Could you check a few things on this model? Use its own coordinates, in mm. Give positions to 0.01 mm unless a question says otherwise; leave off trailing zeros. Loops run counter-clockwise (first coordinate to the right, second up) from the corner with the lowest first, then second, coordinate; pieces in that order, holes last. Notation, with made-up numbers: M 12.5,-18.75 L 69.5,-18.75 A29 cw 69.5,1.25 Z; hole C -36.5,85 d3. An arc over 180 degrees is marked long. Return JSON: item names as keys, results as strings. Group by question number.
1. Please list where these lines run through material, in increasing order: line 1 (X direction, y = 2.35, z = 66); line 2 (X direction, y = 1.45, z = -13.5); line 3 (X direction, y = 1.45, z = 0).
2. If we section it at A-A (z = 30): Write out the boundary of the cut face in (x, y).
3. If we section it at C-C (y = 2.3): State how many separate pieces and enclosed holes the cut face has, plus the area to 3 significant figures.
4. For pin 1 (2.5 mm diameter, centred on x = 90, z = 0, fed in from +Y), with a flat end and sliding along its axis, tell me the tip position at first contact or that it passes through.
5. If we section it at B-B (x = -63.64): Write out the boundary of the cut face in (y, z), plus the area to 3 significant figures.
```python
from build123d import *

# Parameters (mm, degrees)
SKETCH_1_W          = 200
SKETCH_1_H          = 200
SKETCH_1_R          = 2
EXTRUDE_1_DEPTH     = 3
FILLET_1_R          = 25
CUT_EXTRUDE_1_DEPTH = 3


with BuildPart() as part:
    # Эскиз1 → Бобышка-Вытянуть1 (new body)
    with BuildSketch(Plane(origin=(0, 0, 0), x_dir=(1, 0, 0), z_dir=(0, 1, 0))):
        Rectangle(SKETCH_1_W, SKETCH_1_H)
        with Locations(Location((-90, 0, 0), (0, 0, 270))):
            Circle(SKETCH_1_R, mode=Mode.SUBTRACT)
        with Locations(Location((0, 90, 0), (0, 0, 270))):
            Circle(SKETCH_1_R, mode=Mode.SUBTRACT)
        with Locations(Location((90, 0, 0), (0, 0, 270))):
            Circle(SKETCH_1_R, mode=Mode.SUBTRACT)
        with Locations(Location((0, -90, 0), (0, 0, 270))):
            Circle(SKETCH_1_R, mode=Mode.SUBTRACT)
        with BuildLine():
            Line((-66.14, -76.211231978), (-66.14, 76.211231978))
            ThreePointArc((-66.14, 76.211231978), (-63.64, 78.711231978), (-61.14, 76.211231978))
            Line((-61.14, 76.211231978), (-61.14, -76.211231978))
            ThreePointArc((-61.14, -76.211231978), (-63.64, -78.711231978), (-66.14, -76.211231978))
        make_face(mode=Mode.SUBTRACT)
        with BuildLine():
            Line((66.14, -76.211231978), (66.14, 76.211231978))
            ThreePointArc((66.14, 76.211231978), (63.64, 78.711231978), (61.14, 76.211231978))
            Line((61.14, 76.211231978), (61.14, -76.211231978))
            ThreePointArc((61.14, -76.211231978), (63.64, -78.711231978), (66.14, -76.211231978))
        make_face(mode=Mode.SUBTRACT)
        with BuildLine():
            Line((1.5, 76.211231978), (1.5, 23.747339046))
            ThreePointArc((1.5, 23.747339046), (0, 22.247339046), (-1.5, 23.747339046))
            Line((-1.5, 23.747339046), (-1.5, 76.211231978))
            ThreePointArc((-1.5, 76.211231978), (0, 77.711231978), (1.5, 76.211231978))
        make_face(mode=Mode.SUBTRACT)
        with BuildLine():
            Line((1.5, -76.211231978), (1.5, -23.747339046))
            ThreePointArc((1.5, -23.747339046), (0, -22.247339046), (-1.5, -23.747339046))
            Line((-1.5, -23.747339046), (-1.5, -76.211231978))
            ThreePointArc((-1.5, -76.211231978), (0, -77.711231978), (1.5, -76.211231978))
        make_face(mode=Mode.SUBTRACT)
        with BuildLine():
            Line((-1.5, -9.644775033), (-1.5, 9.644775033))
            ThreePointArc((-1.5, 9.644775033), (0, 11.144775033), (1.5, 9.644775033))
            Line((1.5, 9.644775033), (1.5, -9.644775033))
            ThreePointArc((1.5, -9.644775033), (0, -11.144775033), (-1.5, -9.644775033))
        make_face(mode=Mode.SUBTRACT)
    extrude(amount=EXTRUDE_1_DEPTH)

    # Скругление1
    fillet_1_edges = [part.edges().sort_by_distance(p)[0] for p in [
        (100, 1.5, 100),
        (-100, 1.5, 100),
        (-100, 1.5, -100),
        (100, 1.5, -100),
    ]]
    fillet(fillet_1_edges, radius=FILLET_1_R)

    # Эскиз2 → Вырез-Вытянуть1 (cut)
    with BuildSketch(Plane(origin=(0, 3, 0), x_dir=(1, 0, 0), z_dir=(0, 1, 0))):
        with BuildLine():
            Line((51.61254098, 2.5), (75.66745902, 2.5))
            ThreePointArc((75.66745902, 2.5), (78.16745902, 0), (75.66745902, -2.5))
            Line((75.66745902, -2.5), (51.61254098, -2.5))
            ThreePointArc((51.61254098, -2.5), (49.11254098, 0), (51.61254098, 2.5))
        make_face()
        with BuildLine():
            Line((-51.61254098, 2.5), (-75.66745902, 2.5))
            ThreePointArc((-75.66745902, 2.5), (-78.16745902, 0), (-75.66745902, -2.5))
            Line((-75.66745902, -2.5), (-51.61254098, -2.5))
            ThreePointArc((-51.61254098, -2.5), (-49.11254098, 0), (-51.61254098, 2.5))
        make_face()
        with BuildLine():
            Line((-11.396089986, 1.5), (11.396089986, 1.5))
            ThreePointArc((11.396089986, 1.5), (12.896089986, 0), (11.396089986, -1.5))
            Line((11.396089986, -1.5), (-11.396089986, -1.5))
            ThreePointArc((-11.396089986, -1.5), (-12.896089986, 0), (-11.396089986, 1.5))
        make_face()
    extrude(amount=-CUT_EXTRUDE_1_DEPTH, mode=Mode.SUBTRACT)


solid = part.part
```
Answer:
{
 "1": {"line 1": "x = -100 to -66.14, -61.14 to -1.5, 1.5 to 61.14, 66.14 to 100", "line 2": "x = -100 to -66.14, -61.14 to 61.14, 66.14 to 100", "line 3": "x = -100 to -92, -88 to -78.17, -49.11 to -12.9, 12.9 to 49.11, 78.17 to 88, 92 to 100"},
 "2": {"outline": "M -100,0 L -66.14,0 L -66.14,3 L -100,3 Z; M -61.14,0 L -1.5,0 L -1.5,3 L -61.14,3 Z; M 1.5,0 L 61.14,0 L 61.14,3 L 1.5,3 Z; M 66.14,0 L 100,0 L 100,3 L 66.14,3 Z"},
 "3": {"separate pieces": "1", "enclosed holes": "9", "area": "37,200 mm²"},
 "4": {"pin 1": "passes through"},
 "5": {"outline": "M 0,-100 L 3,-100 L 3,-78.71 L 0,-78.71 Z; M 0,78.71 L 3,78.71 L 3,100 L 0,100 Z", "area": "128 mm²"}
}
